Geometry check sheet. Reference: the model listing, model coordinates, mm. A direction names the side the tool comes from. Round coordinates to 2 decimals unless told otherwise and drop trailing zeros. Write each loop counter-clockwise with the first axis right and the second up, starting at its lowest first coordinate (ties: lowest second). Pieces come first, ordered by that corner, then holes. Notation, with made-up numbers: M -7.75,81 L 20.25,81 A18 cw 20.25,109 Z; hole C 61.25,-9 d4. An arc over 180 degrees is marked long. One line per item, written item: value. Start each with the question number.
1. Access from +Z, -Z, +X, -X, +Y, -Y to the whole of each face (thin tool, end or side, straight path). Record for faces 1 (the flat face through (-1.33, 2.48, 1.48)), 2 (the flat face through (-0.25, 2, 1)), 3 (the flat face through (1.33, -2.48, 1.48)), 4 (the flat face through (0.25, -2, 1)).
2. Section check A-A (y = -2.25). Record the boundary of the cut face in (x, z).
3. Depth check by flat-ended pin: P1, Ø1.1, axis at y = 0.5, z = 1, coming from the +X side; P2, Ø0.9, axis at y = -1.5, z = 1.5, coming from the -X side; P3, Ø0.9, axis at y = 2.5, z = 2, coming from the +X side. Enter the tip coordinate at first touch or a pass-through.
4. Release check for a two-part mould opening along Y. For faces 5 (the cylindrical face through (-1.48, 1.5, 1.52)), 6 (the flat face through (0, 0, 3)) record: pulls with the +Y half, pulls with the -Y half, needs draft (parallel to the pull), parting line crosses it, or undercut.
5. Section check C-C (x = 0.1). Record the boundary of the cut face in (y, z).
6. Section check B-B (y = 1.25). Record the boundary of the cut face in (x, z), and give its area (3 significant figures).
7. Scan lines: probe 1 along X at (y, z) = (-0.75, 0.4); probe 2 along Y at (x, z) = (1.55, 0.15); probe 3 along X at (y, z) = (2.5, 0.7). Record each from-to range of solid material in increasing order. Write a range as [from, to].
from build123d import *

# Parameters (mm, degrees)
F1_DEPTH = 3
F2_R     = 0.24999
F3_R     = 5


# Not quite as in the source:
# - a fillet or chamfer is up to 0.001 mm smaller than in the source, because OpenCascade refuses the exact size


with BuildPart() as f1:
    # F0 (on Top) → F1 (new body)
    with BuildSketch(Plane.XY):
        with BuildLine():
            Line((-1.5, 1.5121936516), (-1.5, 0))
            Line((-1.5, 0), (-1.5, -1.5121936516))
            Line((-1.5, -1.5121936516), (-1.2376595987, -3))
            Line((-1.2376595987, -3), (-1.5982141028, -3))
            ThreePointArc((-1.5982141028, -3), (-1.8792268389, -3.1949674233), (-1.7949840479, -3.5264543855))
            Line((-1.7949840479, -3.5264543855), (-1.25, -4))
            Line((-1.25, -4), (-0.25, -4))
            Line((-0.25, -4), (-0.25, -0.4752505826))
            Line((-0.25, -0.4752505826), (0, -0.4752505826))
            Line((0, -0.4752505826), (0.25, -0.4752505826))
            Line((0.25, -0.4752505826), (0.25, -4))
            Line((0.25, -4), (1.25, -4))
            Line((1.25, -4), (1.7949840479, -3.5264543855))
            ThreePointArc((1.7949840479, -3.5264543855), (1.8792268389, -3.1949674233), (1.5982141028, -3))
            Line((1.5982141028, -3), (1.2376595987, -3))
            Line((1.2376595987, -3), (1.5, -1.5121936516))
            Line((1.5, -1.5121936516), (1.5, 1.5121936516))
            Line((1.5, 1.5121936516), (1.2376595987, 3))
            Line((1.2376595987, 3), (1.5982141028, 3))
            ThreePointArc((1.5982141028, 3), (1.8792268389, 3.1949674233), (1.7949840479, 3.5264543855))
            Line((1.7949840479, 3.5264543855), (1.25, 4))
            Line((1.25, 4), (0.25, 4))
            Line((0.25, 4), (0.25, 0.4752505826))
            Line((0.25, 0.4752505826), (0, 0.4752505826))
            Line((0, 0.4752505826), (-0.25, 0.4752505826))
            Line((-0.25, 0.4752505826), (-0.25, 4))
            Line((-0.25, 4), (-1.25, 4))
            Line((-1.25, 4), (-1.7949840479, 3.5264543855))
            ThreePointArc((-1.7949840479, 3.5264543855), (-1.8792268389, 3.1949674233), (-1.5982141028, 3))
            Line((-1.5982141028, 3), (-1.2376595987, 3))
            Line((-1.2376595987, 3), (-1.5, 1.5121936516))
        make_face()
    extrude(amount=F1_DEPTH)

    # F2 (radius 0.25 in the source; OpenCascade refuses exactly that, so slightly less here)
    f2_edges = [f1.edges().sort_by_distance(p)[0] for p in [
        (-1.25, 4, 1.5),
        (-0.25, 4, 1.5),
        (0.25, 4, 1.5),
        (1.25, 4, 1.5),
        (-0.25, 0.475251, 1.5),
        (0.25, 0.475251, 1.5),
        (-0.25, -0.475251, 1.5),
        (0.25, -0.475251, 1.5),
        (-1.25, -4, 1.5),
        (-0.25, -4, 1.5),
        (0.25, -4, 1.5),
        (1.25, -4, 1.5),
    ]]
    fillet(f2_edges, radius=F2_R)

    # F3
    f3_edges = [f1.edges().sort_by_distance(p)[0] for p in [
        (-1.5, -1.512194, 1.5),
        (-1.5, 1.512194, 1.5),
        (1.5, -1.512194, 1.5),
        (1.5, 1.512194, 1.5),
    ]]
    fillet(f3_edges, radius=F3_R)


solid = f1.part
Result sheet:
1. face 1: +Z, -Z, -X
1. face 2: +Z, -Z, +Y
1. face 3: +Z, -Z, +X
1. face 4: +Z, -Z, -Y
2. outline: M -1.37,0 L -0.25,0 L -0.25,3 L -1.37,3 Z; M 0.25,0 L 1.37,0 L 1.37,3 L 0.25,3 Z
3. P1: stops at x = 1.5
3. P2: stops at x = -1.5
3. P3: stops at x = 1.41
4. face 5: undercut
4. face 6: needs draft
5. outline: M -0.5,0 L 0.5,0 L 0.5,3 L -0.5,3 Z
6. outline: M -1.5,0 L -0.25,0 L -0.25,3 L -1.5,3 Z; M 0.25,0 L 1.5,0 L 1.5,3 L 0.25,3 Z
6. area: 7.48 mm2
7. probe 1: x = [-1.5, -0.25], [0.25, 1.5]
7. probe 2: y = [-3.74, -3], [3, 3.74]
7. probe 3: x = [-1.33, -0.25], [0.25, 1.33]
